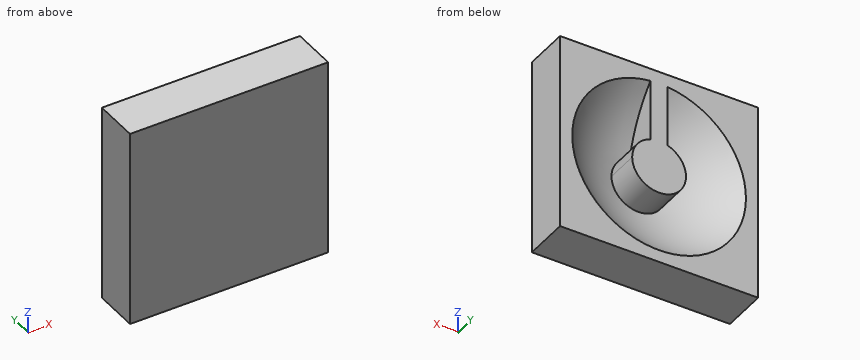
from build123d import *

# Parameters (mm, degrees)
F3_R     = 300
F4_DEPTH = 500
F6_DEPTH = 600
F7_W     = 460
F7_H     = 460
F8_DEPTH = 105


with BuildPart() as f1:
    # F0 (on Front) → F1 (revolve)
    with BuildSketch(Plane.XZ):
        with BuildLine():
            Line((-284, 0), (284, 0))
            ThreePointArc((284, 0), (0, 284), (-284, 0))
        make_face()
    revolve(axis=Axis((0, 0, 0), (1, 0, 0)))

    # F3 (on offset) → F4 (cut)
    with BuildSketch(Plane.XZ.offset(200)):
        Circle(F3_R)
    extrude(amount=-F4_DEPTH, mode=Mode.SUBTRACT)

    # F5 (on Front) → F6 (cut)
    with BuildSketch(Plane.XZ):
        with BuildLine():
            ThreePointArc((-20, 59.213596), (0, 62.5), (20, 59.213596))
            Line((20, 59.213596), (20, 224.58975))
            Line((20, 224.58975), (-20, 224.58975))
            Line((-20, 224.58975), (-20, 59.213596))
        make_face()
        with BuildLine():
            ThreePointArc((-20, 59.213596), (-36.443449, -50.77524), (62.5, 0))
            ThreePointArc((62.5, 0), (50.77524, 36.443449), (20, 59.213596))
            Line((20, 59.213596), (20, 25.99727))
            Line((20, 25.99727), (-20, 25.99727))
            Line((-20, 25.99727), (-20, 59.213596))
        make_face()
        with BuildLine():
            Line((20, 25.99727), (20, 59.213596))
            ThreePointArc((20, 59.213596), (0, 62.5), (-20, 59.213596))
            Line((-20, 59.213596), (-20, 25.99727))
            Line((-20, 25.99727), (20, 25.99727))
        make_face()
    extrude(amount=F6_DEPTH, mode=Mode.SUBTRACT)


with BuildPart() as f8:
    # F7 (on offset) → F8 (new body)
    with BuildSketch(Plane.XZ.offset(200)):
        Rectangle(F7_W, F7_H)
    extrude(amount=F8_DEPTH)

    # F9: cut F1
    add(f1.part, mode=Mode.SUBTRACT)


solid = f8.part
Build history of the part. All positions in model axes, mm. Coordinates: 2 decimals unless noted, no trailing zeros. Write each loop counter-clockwise with the first axis right and the second up, starting at its lowest first coordinate (ties: lowest second). Pieces come first, ordered by that corner, then holes.
(1) Drill centre lines: line 1 (Z direction, x = -43.5, y = -208); line 2 (Z direction, x = 38, y = -212); line 3 (X direction, y = -210, z = 95.5). Where is each one in solid material? Low to high.
(2) Cut at D-D on y = -254. List the corners of the cut face in (x, z).
(3) Pin check, flat tips, straight feed: pin 1 Ø6 at (x, z) = (-139, -2) entering from +Y; pin 2 Ø12 at (x, z) = (166, -102.5) entering from +Y. Stop position of each tip, or through.
(4) Cut at A-A on x = 0. List the corners of the cut face in (y, z).
(5) Cut at C-C on z = -190. List the corners of the cut face in (x, y).
(6) Cut at B-B on y = -228.5. List the corners of the cut face in (x, z).
Working result:
1. line 1: z = -230 to -188.41, -44.88 to 44.88, 188.41 to 230
1. line 2: z = -230 to -185.12, -49.62 to 49.62, 185.12 to 230
1. line 3: x = -230 to -165.64, -20 to 20, 165.64 to 230
2. outline: (-230, -230) - (230, -230) - (230, 230) - (-230, 230) - close; hole (-20, 59.21) - (-20, 125.46) arc R127.04 ccw (long way) to (20, 125.46) - (20, 59.21) arc R62.5 cw (long way) to start
3. pin 1: stops at y = -245.94
3. pin 2: stops at y = -200.54
4. outline: (-305, -230) - (-200, -230) - (-200, -201.63) arc R284 cw to (-277.04, -62.5) - (-200, -62.5) - (-200, 230) - (-305, 230) - close
5. outline: (-230, -305) - (230, -305) - (230, -200) - (67.5, -200) arc R211.08 cw to (-67.5, -200) - (-230, -200) - close
6. outline: (-230, -230) - (230, -230) - (230, 230) - (-230, 230) - close; hole (-20, 59.21) - (-20, 167.46) arc R168.65 ccw (long way) to (20, 167.46) - (20, 59.21) arc R62.5 cw (long way) to start
